For this review, take the finished solid that the model builds, in its own axes (mm). Coordinates: 2 decimals unless noted, no trailing zeros. Write each loop counter-clockwise with the first axis right and the second up, starting at its lowest first coordinate (ties: lowest second). Pieces come first, ordered by that corner, then holes. Notation, with made-up numbers: M 20,-24 L 68,-24 A22 cw 68,-11 Z; hole C 35.5,14.5 d7. An arc over 180 degrees is marked long. One line per question, with ' | ' between items.
from build123d import *

# Parameters (mm, degrees)
F0_W     = 23.7
F0_H     = 13.6
F0_R     = 3.3
F1_DEPTH = 13.6
F2_R     = 3.3
F3_DEPTH = 13.601
F4_R     = 5


with BuildPart() as f1:
    # F0 (on Front) → F1 (new body)
    with BuildSketch(Plane.XZ):
        with Locations((-10.017435, 24.03643)):
            Rectangle(F0_W, F0_H)
        with Locations((-15.067435, 24.03643)):
            Circle(F0_R, mode=Mode.SUBTRACT)
    extrude(amount=F1_DEPTH)

    # F2 (on face) → F3 (cut, through all)
    with BuildSketch(Plane.XY.offset(30.83643)):
        with Locations((-4.967435, -6.8)):
            Circle(F2_R)
    extrude(amount=-F3_DEPTH, mode=Mode.SUBTRACT)

    # F4
    f4_edges = [f1.edges().sort_by_distance(p)[0] for p in [
        (1.832565, -13.6, 24.03643),
        (1.832565, 0, 24.03643),
        (-21.867435, -6.8, 30.83643),
        (-21.867435, -6.8, 17.23643),
    ]]
    fillet(f4_edges, radius=F4_R)


solid = f1.part
1. Clearance check with flat-ended pins moving along their axes: P1, Ø1, axis at x = -2, z = 21, coming from the -Y side; P2, Ø4, axis at x = -2.5, y = -8.5, coming from the -Z side; P3, Ø1, axis at y = -3.5, z = 22.5, coming from the +X side; P4, Ø2, axis at y = -2.5, z = 19.5, coming from the -X side. State where each tip first meets the part, or that it passes through.
Computed values:
P1: stops at y = -13.56 | P2: stops at z = 17.24 | P3: stops at x = 1.73 | P4: stops at x = -21.56
2. Draft analysis for pull direction X (two halves, no side actions). For faces 1 (the cylindrical face through (-20.4, -6.9, 18.7)), 2 (the flat face through (-10, -7, 17.236)), 3 (the cylindrical face through (-17.5, -6.705, 26.267)), 4 (the cylindrical face through (-7.4, -4.57, 24.13)), state which applies: pulls with the +X half, pulls with the -X half, needs draft (parallel to the pull), parting line crosses it, or undercut.
Computed values:
face 1: pulls with the -X half | face 2: needs draft | face 3: undercut | face 4: undercut
3. Take a section at D-D on y = -2.75. State the section outline as (x, z) points.
Computed values:
outline: M -21.87,22.24 A5 ccw -16.87,17.24 L 1.3,17.24 L 1.3,30.84 L -16.87,30.84 A5 ccw -21.87,25.84 Z; hole C -15.07,24.04 d6.6
4. Take a section at C-C on x = -4.25. State the section outline as (y, z) points, plus the area to 3 significant figures.
Computed values:
outline: M -13.6,17.24 L -10.02,17.24 L -10.02,30.84 L -13.6,30.84 Z; M -3.58,17.24 L 0,17.24 L 0,30.84 L -3.58,30.84 Z | area: 97.3 mm2
5. For line 1 along Z through (x, y) = (-15.25, -4.5); line 2 along X through (y, z) = (-5.25, 24.75); line 3 along Z through (x, y) = (-15.5, -9.5), list the stretches that pass through material, from the lowest coordinate up.
Computed values:
line 1: z = 17.24 to 20.74, 27.33 to 30.84 | line 2: x = -21.87 to -18.29, -11.85 to -7.88, -2.05 to 1.83 | line 3: z = 17.24 to 20.76, 27.31 to 30.84
6. Take a section at A-A on y = -6.8. State the section outline as (x, z) points.
Computed values:
outline: M -21.87,22.24 A5 ccw -16.87,17.24 L -8.27,17.24 L -8.27,30.84 L -16.87,30.84 A5 ccw -21.87,25.84 Z; M -1.67,17.24 L 1.83,17.24 L 1.83,30.84 L -1.67,30.84 Z; hole C -15.07,24.04 d6.6
7. Take a section at B-B on z = 22.75. State the section outline as (x, y) points.
Computed values:
outline: M -21.87,-13.6 L -18.11,-13.6 L -18.11,0 L -21.87,0 Z; M -12.03,-13.6 L -3.17,-13.6 A5 ccw 1.83,-8.6 L 1.83,-5 A5 ccw -3.17,0 L -12.03,0 Z; hole C -4.97,-6.8 d6.6
